from build123d import *

# Parameters (mm, degrees)
SKETCH1_R                        = 6
BOSS_EXTRUDE1_DEPTH              = 19
M24X2_0_TAPPED_HOLE1_D           = 22
M24X2_0_TAPPED_HOLE1_DEPTH       = 38
M24X2_0_TAPPED_HOLE1_CSINK_D     = 24.05
M24X2_0_TAPPED_HOLE1_CSINK_ANGLE = 100
M24X2_0_TAPPED_HOLE1_TIP         = 6.609466809


with BuildPart() as part:
    # Sketch1 → Boss-Extrude1 (new, symmetric)
    with BuildSketch(Plane(origin=(0, 0, 0), x_dir=(1, 0, 0), z_dir=(0, 1, 0))):
        with BuildLine():
            Line((-19, 0), (-19, 70))
            ThreePointArc((-19, 70), (0, 89), (19, 70))
            Line((19, 70), (19, 0))
            ThreePointArc((19, 0), (0, -19), (-19, 0))
        make_face()
        with Locations(Location((0, 70, 0), (0, 0, 270))):
            Circle(SKETCH1_R, mode=Mode.SUBTRACT)
        with Locations(Location((0, 0, 0), (0, 0, 270))):
            Circle(SKETCH1_R, mode=Mode.SUBTRACT)
    extrude(amount=BOSS_EXTRUDE1_DEPTH, both=True)

    # M24x2.0 Tapped Hole1
    with Locations(Plane(origin=(19, 0, 0), x_dir=(0, 0, -1), z_dir=(1, 0, 0))):
        with Locations((35, 0)):
            CounterSinkHole(M24X2_0_TAPPED_HOLE1_D / 2, M24X2_0_TAPPED_HOLE1_CSINK_D / 2, depth=M24X2_0_TAPPED_HOLE1_DEPTH, counter_sink_angle=M24X2_0_TAPPED_HOLE1_CSINK_ANGLE)
            with Locations((0, 0, -(M24X2_0_TAPPED_HOLE1_DEPTH + M24X2_0_TAPPED_HOLE1_TIP / 2))):  # 118° drill point
                Cone(0, M24X2_0_TAPPED_HOLE1_D / 2, M24X2_0_TAPPED_HOLE1_TIP, mode=Mode.SUBTRACT)


solid = part.part
Here's how the part is built. I have some questions about the finished solid (model axes, mm). Round coordinates to 2 decimals unless told otherwise and drop trailing zeros. Order: outer loops, then holes, each group sorted by start corner. A loop starts at its lowest first (then second) coordinate and runs counter-clockwise, first axis right, second up. Notation, with made-up numbers: (76.25, 57) -> (92.25, 57) arc R36 ccw to (92.25, 93) -> close; hole circle Ø5 at (-8, 60.25). An arc over 180 degrees is marked (long way). Return JSON: item names as keys, results as strings.
Q1. If we section it at B-B on z = -35: List the corners of the cut face in (x, y) for me (3 decimals), plus the area to 3 significant figures.
Filled sheet:
{"outline": "(-19, -19) -> (19, -19) -> (19, -12.025) -> (18.14, -11) -> (-19, -11) -> close; (-19, 11) -> (18.14, 11) -> (19, 12.025) -> (19, 19) -> (-19, 19) -> close", "area": "607 mm^2"}
Q2. If we mould it in two halves opening along Z, with no side actions, what happens to faces 1 (the cylindrical face through (0, 0, -76)), 2 (the flat face through (0, -19, -36)), 3 (the cylindrical face through (0, 0, -89))? For each: released by +Z, released by -Z, zero draft, split by the parting line, or undercut.
Filled sheet:
{"face 1": "undercut", "face 2": "zero draft", "face 3": "released by -Z"}
Q3. For pin 1 Ø3 at (x, y) = (9, 6) entering from -Z; pin 2 Ø4 at (x, y) = (-2, -14.5) entering from -Z; pin 3 Ø4 at (x, y) = (11.5, 4.5) entering from -Z, each with a flat end and sliding along its axis, tell me the tip position at first contact or that it passes through.
Filled sheet:
{"pin 1": "stops at z = -87.46", "pin 2": "stops at z = -89", "pin 3": "stops at z = -86.45"}
Q4. If we section it at A-A on x = 0: List the corners of the cut face in (y, z) for me, plus the area to 3 significant figures.
Filled sheet:
{"outline": "(-19, -89) -> (19, -89) -> (19, -76) -> (-19, -76) -> close; (-19, -64) -> (19, -64) -> (19, -6) -> (-19, -6) -> close; (-19, 6) -> (19, 6) -> (19, 19) -> (-19, 19) -> close; hole circle Ø22 at (0, -35)", "area": "2,810 mm^2"}
Q5. If we section it at D-D on x = -15.5: List the corners of the cut face in (y, z) for me, plus the area to 4 significant figures.
Filled sheet:
{"outline": "(-19, -80.99) -> (19, -80.99) -> (19, 10.99) -> (-19, 10.99) -> close; hole circle Ø22 at (0, -35)", "area": "3,115 mm^2"}
Q6. I need wall thicknesses on line 1 along X through (y, z) = (10.5, -70); line 2 along Y through (x, z) = (-3, -35); line 3 along Z through (x, y) = (8, -1.5). Which ranges of each line are inside material? Lowest first, please. Write a range as from..to.
Filled sheet:
{"line 1": "x = -19..-6, 6..19", "line 2": "y = -19..-11, 11..19", "line 3": "z = -87.23..-45.9, -24.1..17.23"}
Q7. If we section it at C-C on y = 15.5: List the corners of the cut face in (x, z) for me.
Filled sheet:
{"outline": "(-19, -70) arc R19 ccw to (19, -70) -> (19, 0) arc R19 ccw to (-19, 0) -> close; hole circle Ø12 at (0, -70); hole circle Ø12 at (0, 0)"}
